```python
from build123d import *

# Parameters (mm, degrees)
SKETCH_1_W          = 80
SKETCH_1_H          = 45
EXTRUDE_1_DEPTH     = 5
SKETCH_2_R          = 1.65
SKETCH_2_R_2        = 4
SKETCH_2_R_3        = 11
CUT_EXTRUDE_1_DEPTH = 47.165463282
SKETCH_3_R          = 7.5
SKETCH_3_R_2        = 4
EXTRUDE_2_DEPTH     = 10
EXTRUDE_4_DEPTH     = 5


with BuildPart() as part:
    # 草图1 → 凸台-拉伸1 (new body)
    with BuildSketch(Plane(origin=(0, 0, 0), x_dir=(1, 0, 0), z_dir=(0, 1, 0))):
        Rectangle(SKETCH_1_W, SKETCH_1_H)
    extrude(amount=EXTRUDE_1_DEPTH)

    # 草图2 → 切除-拉伸1 (cut, through all)
    with BuildSketch(Plane(origin=(0, 5, 0), x_dir=(1, 0, 0), z_dir=(0, 1, 0))):
        with Locations(Location((-15.5, 15.5, 0), (0, 0, 270))):
            Circle(SKETCH_2_R)
        with Locations(Location((15.5, 15.5, 0), (0, 0, 270))):
            Circle(SKETCH_2_R)
        with Locations(Location((15.5, -15.5, 0), (0, 0, 270))):
            Circle(SKETCH_2_R)
        with Locations(Location((-15.5, -15.5, 0), (0, 0, 270))):
            Circle(SKETCH_2_R)
        with Locations(Location((30, 15.5, 0), (0, 0, 270))):
            Circle(SKETCH_2_R)
        with Locations(Location((30, -15.5, 0), (0, 0, 270))):
            Circle(SKETCH_2_R)
        with Locations(Location((-28, 0, 0), (0, 0, 270))):
            Circle(SKETCH_2_R_2)
        with Locations(Location((0, 0, 0), (0, 0, 270))):
            Circle(SKETCH_2_R_3)
    extrude(amount=-CUT_EXTRUDE_1_DEPTH, mode=Mode.SUBTRACT)

    # 草图3 → 凸台-拉伸2 (add)
    with BuildSketch(Plane.XZ):
        with Locations(Location((-28, 0, 0), (0, 0, 90))):
            Circle(SKETCH_3_R)
        with Locations(Location((-28, 0, 0), (0, 0, 90))):
            Circle(SKETCH_3_R_2, mode=Mode.SUBTRACT)
    extrude(amount=EXTRUDE_2_DEPTH)

    # 草图6 → 凸台-拉伸4 (add)
    with BuildSketch(Plane.XY.offset(22.5)):
        Polygon((-40, 5), (-40, -10), (20, -35), (20, 5), align=None)
    extrude_4 = extrude(amount=EXTRUDE_4_DEPTH)

    # 镜向1: 凸台-拉伸4 across plane
    add(extrude_4.mirror(Plane(origin=(0, 0, 0), x_dir=(1, 0, 0), z_dir=(0, 0, -1))))


solid = part.part
```
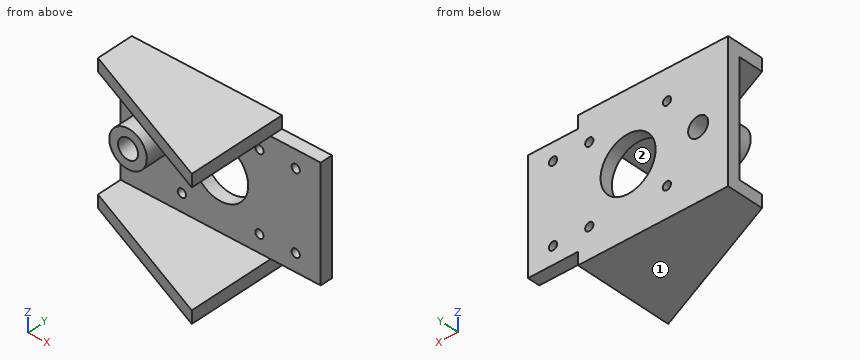
Work out the finished part from the listing and answer in its coordinate system (mm). Face numbers are marked on the shaded views. A direction names the side the tool comes from. Give positions to 0.01 mm unless a question says otherwise; leave off trailing zeros. Order: outer loops, then holes, each group sorted by start corner. A loop starts at its lowest first (then second) coordinate and runs counter-clockwise, first axis right, second up.
1. Section C-C, the plane z = -15.5 is taken. Determine the outline of the cut face in (x, y), and give its area (4 significant figures).
Result sheet:
outline: (-40, 0) - (-17.15, 0) - (-17.15, 5) - (-40, 5) - close; (-13.85, 0) - (13.85, 0) - (13.85, 5) - (-13.85, 5) - close; (17.15, 0) - (28.35, 0) - (28.35, 5) - (17.15, 5) - close; (31.65, 0) - (40, 0) - (40, 5) - (31.65, 5) - close
area: 350.5 mm2
2. Straight lines are drawn through the part: L1, parallel to X at y = 3, z = 0; L2, parallel to X at y = 3.2, z = 15.5; L3, parallel to Z at x = -15, y = 2. For each, find the intervals that lie inside material, in ascending order.
Result sheet:
L1: x = -40 to -32, -24 to -11, 11 to 40
L2: x = -40 to -17.15, -13.85 to 13.85, 17.15 to 28.35, 31.65 to 40
L3: z = -27.5 to -17.07, -13.93 to 13.93, 17.07 to 27.5
3. Section B-B, the plane x = 30 is taken. Determine the outline of the cut face in (y, z).
Result sheet:
outline: (0, -22.5) - (5, -22.5) - (5, -17.15) - (0, -17.15) - close; (0, -13.85) - (5, -13.85) - (5, 13.85) - (0, 13.85) - close; (0, 17.15) - (5, 17.15) - (5, 22.5) - (0, 22.5) - close
4. Section A-A, the plane y = -26 is taken. Determine the outline of the cut face in (x, z).
Result sheet:
outline: (-1.6, -27.5) - (20, -27.5) - (20, -22.5) - (-1.6, -22.5) - close; (-1.6, 22.5) - (20, 22.5) - (20, 27.5) - (-1.6, 27.5) - close
5. Section D-D, the plane y = -12 is taken. Determine the outline of the cut face in (x, z).
Result sheet:
outline: (-35.2, -27.5) - (20, -27.5) - (20, -22.5) - (-35.2, -22.5) - close; (-35.2, 22.5) - (20, 22.5) - (20, 27.5) - (-35.2, 27.5) - close
6. For the marked faces 1 and 2, determine the directions among +Z, -Z, +X, -X, +Y, -Y from which every point of the face is accessible in a straight line to the end or side of a thin tool.
Result sheet:
face 1: -Z, +X, -X, +Y, -Y
face 2: +X, -X, -Y
7. Each of these flat-tipped pins is pushed along its axis until it touches: P1, Ø4.5, axis at x = 30, z = -15.5, coming from the +Y side; P2, Ø3, axis at x = -29.5, z = 20.5, coming from the -Y side; P3, Ø5.5, axis at x = 27, y = 3, coming from the -Z side; P4, Ø1.5, axis at y = -7.5, z = 24.5, coming from the +X side. Where does it stop, or does it pass through?
Result sheet:
P1: stops at y = 5
P2: stops at y = 0
P3: stops at z = -22.5
P4: stops at x = 20
